Here's how the part is built. I have some questions about the finished solid (model axes, mm). Face numbers are marked on the shaded views. Round coordinates to 2 decimals unless told otherwise and drop trailing zeros. Order: outer loops, then holes, each group sorted by start corner. A loop starts at its lowest first (then second) coordinate and runs counter-clockwise, first axis right, second up. Notation, with made-up numbers: M 54,82 L 89,82 A15 cw 89,95 Z; hole C -38.75,81 d9. An arc over 180 degrees is marked long. Write item = value, one per line. Start each with the question number.
Item 1: I'm going to push a flat-ended pin straight in: P1, Ø4.5, axis at x = 39.5, z = 33, coming from the +Y side. Where does the tip first touch, or does it pass through?
Item 2: I want a section at A-A, the plane y = 36. List the corners of the cut face in (x, z) for me.
Item 3: I want a section at D-D, the plane z = -4. List the corners of the cut face in (x, y) for me.
Item 4: We'd pull the mould along Z, two halves only. Please class the marked faces 1, 2 and 3: pulls with the +Z half, pulls with the -Z half, needs draft (parallel to the pull), parting line crosses it, or undercut.
Item 5: I want a section at B-B, the plane x = 14. List the corners of the cut face in (y, z) for me.
Item 6: Please list where these lines run through material, in increasing order: L1, parallel to X at y = 28, z = 25.5; L2, parallel to Z at x = -11, y = 13.5; L3, parallel to Y at x = 29, z = -5.
Item 7: I want a section at C-C, the plane x = 4. List the corners of the cut face in (y, z) for me, plus the area to 4 significant figures.
```python
from build123d import *

# Parameters (mm, degrees)
SKETCH1_W            = 95.5
SKETCH1_H            = 75.5
SKETCH1_W_2          = 91.5
SKETCH1_H_2          = 71.5
EXTRUDE_THIN1_DEPTH  = 40
SKETCH2_W            = 95.5
SKETCH2_H            = 75.5
BOSS_EXTRUDE1_DEPTH  = 3
CUT_EXTRUDE1_DEPTH   = 98.879070797
BOSS_EXTRUDE3_START  = 11
BOSS_EXTRUDE3_DEPTH  = 9
CUT_EXTRUDE2_REACH   = 83.241
MIRROR2_START        = 11
MIRROR2_COPY_1_DEPTH = 9
MIRROR2_COPY_2_REACH = 83.241
FILLET3_R            = 0.75
FILLET4_R            = 0.75


with BuildPart() as part:
    # Sketch1 → Extrude-Thin1 (new body)
    with BuildSketch(Plane(origin=(0, 0, 0), x_dir=(1, 0, 0), z_dir=(0, 1, 0))):
        Rectangle(SKETCH1_W, SKETCH1_H)
        Rectangle(SKETCH1_W_2, SKETCH1_H_2, mode=Mode.SUBTRACT)
    extrude(amount=EXTRUDE_THIN1_DEPTH)

    # Sketch2 → Boss-Extrude1 (add)
    with BuildSketch(Plane.XZ):
        Rectangle(SKETCH2_W, SKETCH2_H)
    extrude(amount=BOSS_EXTRUDE1_DEPTH)

    # Sketch4 → Cut-Extrude1 (cut, through all)
    with BuildSketch(Plane.XY.offset(37.75)):
        with BuildLine():
            Line((-22, 32), (-11, 32))
            ThreePointArc((-11, 32), (-8.525126266, 30.974873734), (-7.5, 28.5))
            Line((-7.5, 28.5), (-7.5, 27.5))
            ThreePointArc((-7.5, 27.5), (-8.525126266, 25.025126266), (-11, 24))
            Line((-11, 24), (-22, 24))
            ThreePointArc((-22, 24), (-24.474873734, 25.025126266), (-25.5, 27.5))
            Line((-25.5, 27.5), (-25.5, 28.5))
            ThreePointArc((-25.5, 28.5), (-24.474873734, 30.974873734), (-22, 32))
        make_face()
        with BuildLine():
            Line((11, 32), (22, 32))
            ThreePointArc((22, 32), (24.474873734, 30.974873734), (25.5, 28.5))
            Line((25.5, 28.5), (25.5, 27.5))
            ThreePointArc((25.5, 27.5), (24.474873734, 25.025126266), (22, 24))
            Line((22, 24), (11, 24))
            ThreePointArc((11, 24), (8.525126266, 25.025126266), (7.5, 27.5))
            Line((7.5, 27.5), (7.5, 28.5))
            ThreePointArc((7.5, 28.5), (8.525126266, 30.974873734), (11, 32))
        make_face()
    extrude(amount=-CUT_EXTRUDE1_DEPTH, mode=Mode.SUBTRACT)

    # Sketch7 → Boss-Extrude3 (add)
    with BuildSketch(Plane(origin=(0, 0, 0), x_dir=(1, 0, 0), z_dir=(0, 1, 0)).offset(BOSS_EXTRUDE3_START)):
        Polygon((-45.75, 35.75), (-45.75, 31.75), (-38.678932188, 24.678932188), (-34.678932188, 28.678932188), (-41.75, 35.75), align=None)
    boss_extrude3 = extrude(amount=-BOSS_EXTRUDE3_DEPTH)

    # Sketch8 → Cut-Extrude2 (cut, up to next)
    with BuildSketch(Plane(origin=(-7, 0, 7), x_dir=(0.7071067811865489, 0, 0.7071067811865461), z_dir=(-0.7071067811865461, 0, 0.7071067811865489)), mode=Mode.PRIVATE) as cut_extrude2_sk1:
        with BuildLine():
            ThreePointArc((-47.300775542, 11), (-45.423796616, 8.62675879), (-46.800775542, 5.932458739))
            Line((-46.800775542, 5.932458739), (-53.550775542, 2))
            Line((-53.550775542, 2), (-44.800775542, 2))
            Line((-44.800775542, 2), (-44.800775542, 11))
            Line((-44.800775542, 11), (-47.300775542, 11))
        make_face()
    cut_extrude2_tool1 = extrude(cut_extrude2_sk1.sketch, amount=-CUT_EXTRUDE2_REACH, mode=Mode.PRIVATE) & part.part
    cut_extrude2 = cut_extrude2_tool1.solids().sort_by_distance((-40.481625, 4.582192, -26.481625))[0]
    add(cut_extrude2, mode=Mode.SUBTRACT)

    # Mirror1: Boss-Extrude3, Cut-Extrude2 across plane
    add(boss_extrude3.mirror(Plane.XY))
    add(cut_extrude2.mirror(Plane.XY), mode=Mode.SUBTRACT)

    # Mirror2: Boss-Extrude3, Cut-Extrude2 across plane
    add(boss_extrude3.mirror(Plane(origin=(0, 0, 0), x_dir=(0, 0, 1), z_dir=(1, 0, 0))))
    add(cut_extrude2.mirror(Plane(origin=(0, 0, 0), x_dir=(0, 0, 1), z_dir=(1, 0, 0))), mode=Mode.SUBTRACT)

    # Mirror2 copy 1 sketch → Mirror2 copy 1 (add)
    with BuildSketch(Plane(origin=(0, 0, 0), x_dir=(-1, 0, 0), z_dir=(0, 1, 0)).offset(MIRROR2_START)):
        Polygon((-45.75, 35.75), (-45.75, 31.75), (-38.678932188, 24.678932188), (-34.678932188, 28.678932188), (-41.75, 35.75), align=None)
    extrude(amount=-MIRROR2_COPY_1_DEPTH)

    # Mirror2 copy 2 sketch → Mirror2 copy 2 (cut, up to next)
    with BuildSketch(Plane(origin=(7, 0, -7), x_dir=(-0.7071067811865489, 0, -0.7071067811865461), z_dir=(0.7071067811865461, 0, -0.7071067811865489)), mode=Mode.PRIVATE) as mirror2_copy_2_sk1:
        with BuildLine():
            ThreePointArc((-47.300775542, 11), (-45.423796616, 8.62675879), (-46.800775542, 5.932458739))
            Line((-46.800775542, 5.932458739), (-53.550775542, 2))
            Line((-53.550775542, 2), (-44.800775542, 2))
            Line((-44.800775542, 2), (-44.800775542, 11))
            Line((-44.800775542, 11), (-47.300775542, 11))
        make_face()
    mirror2_copy_2_tool1 = extrude(mirror2_copy_2_sk1.sketch, amount=-MIRROR2_COPY_2_REACH, mode=Mode.PRIVATE) & part.part
    add(mirror2_copy_2_tool1.solids().sort_by_distance((40.481625, 4.582192, 26.481625))[0], mode=Mode.SUBTRACT)

    # Fillet3
    fillet3_edges = [part.edges().sort_by_distance(p)[0] for p in [
        (-45.75, 0, 0),
        (0, 0, 35.75),
        (45.75, 0, 0),
        (0, 0, -35.75),
        (45.75, 25.5, 35.75),
        (45.75, 25.5, -35.75),
        (-45.75, 25.5, -35.75),
        (-45.75, 25.5, 35.75),
    ]]
    fillet(fillet3_edges, radius=FILLET3_R)

    # Fillet4
    fillet4_edges = [part.edges().sort_by_distance(p)[0] for p in [
        (-45.75, 40, 0),
        (0, 40, 35.75),
        (45.75, 40, 0),
        (0, 40, -35.75),
        (45.530330086, 40, 35.530330086),
        (45.530330086, 40, -35.530330086),
        (-45.530330086, 40, -35.530330086),
        (-45.530330086, 40, 35.530330086),
    ]]
    fillet(fillet4_edges, radius=FILLET4_R)


solid = part.part
```
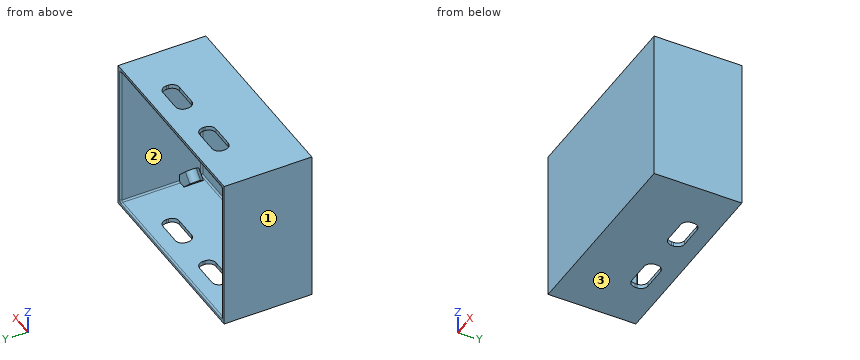
Filled in:
q1.P1 = 11
q2.outline = M -47.75,-37.75 L 47.75,-37.75 L 47.75,37.75 L -47.75,37.75 Z; hole M -45.75,-35 A0.75 ccw -45,-35.75 L 45,-35.75 A0.75 ccw 45.75,-35 L 45.75,35 A0.75 ccw 45,35.75 L -45,35.75 A0.75 ccw -45.75,35 Z
q3.outline = M -47.75,-3 L 47.75,-3 L 47.75,40 L 46.5,40 A0.75 ccw 45.75,39.25 L 45.75,0.75 A0.75 cw 45,0 L -45,0 A0.75 cw -45.75,0.75 L -45.75,39.25 A0.75 ccw -46.5,40 L -47.75,40 Z
q4.face_1 = needs draft
q4.face_2 = undercut
q4.face_3 = pulls with the -Z half
q5.outline = M -3,-37.75 L 24,-37.75 L 24,-35.75 L 0.75,-35.75 A0.75 cw 0,-35 L 0,35 A0.75 cw 0.75,35.75 L 24,35.75 L 24,37.75 L -3,37.75 Z; M 32,-37.75 L 40,-37.75 L 40,-36.5 A0.75 ccw 39.25,-35.75 L 32,-35.75 Z; M 32,35.75 L 39.25,35.75 A0.75 ccw 40,36.5 L 40,37.75 L 32,37.75 Z
q6.L1 = -47.75 to -45.75, 45.75 to 47.75
q6.L2 = -37.75 to -35.75, 35.75 to 37.75
q6.L3 = -3 to 0
q7.outline = M -3,-37.75 L 40,-37.75 L 40,-36.5 A0.75 ccw 39.25,-35.75 L 0.75,-35.75 A0.75 cw 0,-35 L 0,35 A0.75 cw 0.75,35.75 L 39.25,35.75 A0.75 ccw 40,36.5 L 40,37.75 L -3,37.75 Z
q7.area = 386.5 mm^2
